```python
from build123d import *

# Parameters (mm, degrees)
FILLET1_R          = 0.25
SKETCH2_W          = 0.25
SKETCH2_H          = 0.25
CUT_EXTRUDE1_DEPTH = 6.338539126


with BuildPart() as part:
    # Sketch1 → Revolve1 (revolve)
    with BuildSketch(Plane(origin=(0, 0, 0), x_dir=(0, 0, -1), z_dir=(1, 0, 0)), mode=Mode.PRIVATE) as revolve1_sk:
        Polygon((-1, 0.5), (1, 0.5), (1, 0.875), (0.125, 0.875), (0.125, 2.5), (0.75, 2.5), (0.75, 3.5), (0.431985117, 3.5), (0.25, 3), (-0.25, 3), (-0.431985117, 3.5), (-0.75, 3.5), (-0.75, 2.5), (-0.125, 2.5), (-0.125, 0.875), (-1, 0.875), align=None)
    revolve(revolve1_sk.sketch.rotate(Axis((0, 0, 48.379703039), (0, 0, -1)), 90), axis=Axis((0, 0, 48.379703039), (0, 0, -1)))

    # Fillet1
    fillet1_edges = [part.edges().sort_by_distance(p)[0] for p in [
        (-0.875, 0, 0.125),
        (-2.5, 0, 0.125),
        (-2.5, 0, -0.125),
        (-0.875, 0, -0.125),
    ]]
    fillet(fillet1_edges, radius=FILLET1_R)

    # Sketch2 → Cut-Extrude1 (cut, through all)
    with BuildSketch(Plane.XY.offset(1)):
        with Locations((0, 0.475)):
            Rectangle(SKETCH2_W, SKETCH2_H)
    extrude(amount=-CUT_EXTRUDE1_DEPTH, mode=Mode.SUBTRACT)


solid = part.part
```
Build history of the part. All positions in model axes, mm. A direction names the side the tool comes from. Coordinates: 2 decimals unless noted, no trailing zeros. Answer in a Markdown table with one row per item. Add a question column.
Q1. Mould opens along Y. For faces 4 (the face through (0, -0.5, 0)), 5 (the face through (-2, 2, -0.75)), 6 (the face through (2.86, -0.9, 0)) say: +Y half, -Y half, draft (parallel to the pull), parting line (faces both ways), or undercut.
Q2. Wall check: line 1 along Y through (x, z) = (0, 0.6) (3 decimals); line 2 along Y through (x, z) = (0, -0.8) (3 decimals); line 3 along Z through (x, y) = (0.75, 2) (3 decimals). Give the ranges that are in metal, low to high. Write a range as [from, to].
Q3. Which spindle directions (+Z, -Z, +X, -X, +Y, -Y) get a long thin tool onto all of the face, cutting with end or side? Do faces 1 (the face through (-1, -1, 0.125)), 2 (the face through (0.4, 0.78, -0.68)), 3 (the face through (1.615, 3.105, -0.589)). Say none if no direction does.
Q4. Drop a flat-ended pin along its axis: pin 1 (1.3 mm diameter, centred on x = 1, y = 1, fed in from -Z). Give the stop position or say it passes through.
Answers follow:
| question | item | result |
|---|---|---|
| 1 | face 4 | undercut |
| 1 | face 5 | draft |
| 1 | face 6 | parting line |
| 2 | line 1 | [-3.5, -2.5], [-0.875, -0.5], [0.6, 0.875], [2.5, 3.5] |
| 2 | line 2 | [-0.875, -0.5], [0.6, 0.875] |
| 2 | line 3 | [-0.125, 0.125] |
| 3 | face 1 | +Z |
| 3 | face 2 | -Z |
| 3 | face 3 | +Z, -Z |
| 4 | pin 1 | z = -1 |
